```python
from build123d import *

# Parameters (mm, degrees)
ESQUISSE1_R             = 24.5
ESQUISSE1_R_2           = 1.5
BOSS_EXTRU_1_DEPTH      = 8
ESQUISSE2_OUTSIDE_W     = 64.952
ESQUISSE2_OUTSIDE_H     = 64.952
ESQUISSE2_OUTSIDE_R     = 24.1
ENL_V_MAT_EXTRU_1_DEPTH = 1.5
CHANFREIN1_SIZE         = 0.5


with BuildPart() as part:
    # Esquisse1 → Boss.-Extru.1 (new body)
    with BuildSketch(Plane(origin=(0, 0, 0), x_dir=(1, 0, 0), z_dir=(0, 1, 0))):
        Circle(ESQUISSE1_R)
        with Locations((0, 15)):
            Circle(ESQUISSE1_R_2, mode=Mode.SUBTRACT)
        with Locations((15, 0)):
            Circle(ESQUISSE1_R_2, mode=Mode.SUBTRACT)
        with Locations((0, -15)):
            Circle(ESQUISSE1_R_2, mode=Mode.SUBTRACT)
        with Locations((-15, 0)):
            Circle(ESQUISSE1_R_2, mode=Mode.SUBTRACT)
    extrude(amount=BOSS_EXTRU_1_DEPTH)

    # Esquisse2 outside → Enlèv. mat.-Extru.1 (cut)
    with BuildSketch(Plane(origin=(0, 8, 0), x_dir=(1, 0, 0), z_dir=(0, 1, 0))):
        Rectangle(ESQUISSE2_OUTSIDE_W, ESQUISSE2_OUTSIDE_H)
        Circle(ESQUISSE2_OUTSIDE_R, mode=Mode.SUBTRACT)
    extrude(amount=-ENL_V_MAT_EXTRU_1_DEPTH, mode=Mode.SUBTRACT)

    # Chanfrein1
    chanfrein1_edges = [part.edges().sort_by_distance(p)[0] for p in [
        (-24.5, 0, 0),
    ]]
    chamfer(chanfrein1_edges, length=CHANFREIN1_SIZE)


solid = part.part
```
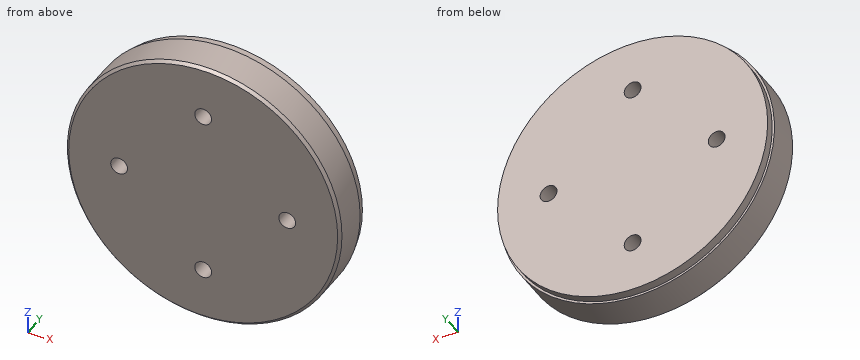
Here's how the part is built. I have some questions about the finished solid (model axes, mm). Round coordinates to 2 decimals unless told otherwise and drop trailing zeros. Loops run counter-clockwise (first coordinate to the right, second up) from the corner with the lowest first, then second, coordinate; pieces in that order, holes last. Notation, with made-up numbers: (40.25, 0) -> (73.25, 0) arc R23 cw to (73.25, 29) -> close; hole circle Ø3 at (56, -1.75). An arc over 180 degrees is marked (long way). Answer as CSV lines item,"result". Start each with the question number.
1. Imagine slicing it at B-B on z = 0. Write out the boundary of the cut face in (x, y).
2. I need wall thicknesses on probe 1 along X at (y, z) = (2.5, 0); probe 2 along Z at (x, y) = (15, 6.25). Which ranges of each line are inside material? Lowest first, please. Write a range as from..to.
3. I'm going to push flat-ended pins straight in: P1, Ø1.8, axis at x = 0, z = -15, coming from the +Y side; P2, Ø4, axis at x = -5, y = 5.5, coming from the +Z side; P3, Ø1.5, axis at x = 18.5, y = 6, coming from the +Z side; P4, Ø4, axis at y = 4, z = 19, coming from the -X side. Where does each tip first touch, or does it pass through?
4. Imagine slicing it at A-A on y = 4.5. Write out the boundary of the cut face in (x, z), plus the area to 3 significant figures.
Solution:
1,outline,"(-24.5, 0.5) -> (-24, 0) -> (-16.5, 0) -> (-16.5, 8) -> (-24.1, 8) -> (-24.1, 6.5) -> (-24.5, 6.5) -> close; (-13.5, 0) -> (13.5, 0) -> (13.5, 8) -> (-13.5, 8) -> close; (16.5, 0) -> (24, 0) -> (24.5, 0.5) -> (24.5, 6.5) -> (24.1, 6.5) -> (24.1, 8) -> (16.5, 8) -> close"
2,probe 1,"-24.5..-16.5, -13.5..13.5, 16.5..24.5"
2,probe 2,"-19.37..-1.5, 1.5..19.37"
3,P1,"through"
3,P2,"z = 24.32"
3,P3,"z = 16.89"
3,P4,"x = -17.64"
4,outline,"circle Ø49 at (0, 0); hole circle Ø3 at (-15, 0); hole circle Ø3 at (0, -15); hole circle Ø3 at (0, 15); hole circle Ø3 at (15, 0)"
4,area,"1,860 mm²"
